Can you work these out from the model? Positions are in its coordinate system, mm. Give positions to 0.01 mm unless a question says otherwise; leave off trailing zeros. Loops run counter-clockwise (first coordinate to the right, second up) from the corner with the lowest first, then second, coordinate; pieces in that order, holes last.
from build123d import *

# Parameters (mm, degrees)
F1_DEPTH    = 86.19552
F3_DEPTH    = 86.19652
F4_T1_DEPTH = 131.920043526


# Not quite as in the source:
# - a fillet or chamfer that OpenCascade refuses, or shapes differently, is made with other operations: its cross-section is extruded or revolved along the edge and cut away or added


with BuildPart() as f1:
    # F0 (on Front) → F1 (new body)
    with BuildSketch(Plane.XZ):
        Polygon((7.1333632804, 110.441185534), (0, 110.441185534), (0, 0), (62.41620332, 0), (62.41620332, 7.1333632804), (7.1333632804, 7.1333632804), align=None)
    extrude(amount=-F1_DEPTH)

    # F2 (on face) → F3 (cut, through all)
    with BuildSketch(Plane.XZ):
        Polygon((7.1333632804, 110.441185534), (7.1333632804, 7.1333632804), (25.2087078989, 24.2729913443), (25.2087078989, 110.441185534), align=None)
        Polygon((2.0419980865, 110.441185534), (7.1333632804, 7.1333632804), (7.1333632804, 110.441185534), align=None)
    extrude(amount=-F3_DEPTH, mode=Mode.SUBTRACT)

    # F4: chamfer of 8.89 on 1 edges, made by hand

    # F4_s2 → F4_t1 (cut)
    with BuildSketch(Plane.XZ.offset(-109.057781763)):
        Polygon((53.52620332, 7.1333632804), (62.41620332, -1.7566367196), (62.41620332, 7.1333632804), align=None)
    extrude(amount=F4_T1_DEPTH, mode=Mode.SUBTRACT)


solid = f1.part
(1) Please list where these lines run through material, in increasing order: probe 1 along Z at (x, y) = (38, 59.5); probe 2 along X at (y, z) = (63, 25); probe 3 along X at (y, z) = (28.5, 68).
Returned:
probe 1: z = 0 to 7.13
probe 2: x = 0 to 6.25
probe 3: x = 0 to 4.13
(2) Thinking about a two-plate mould opening in Z: for faces 1 (the flat face through (5, 86.196, 27)), 2 (the flat face through (30, 42, 0)), 3 (the flat face through (31, 42, 7.133)), which applies, pulls with the +Z half, pulls with the -Z half, needs draft (parallel to the pull), parting line crosses it, or undercut?
Returned:
face 1: needs draft
face 2: pulls with the -Z half
face 3: pulls with the +Z half
(3) Suppose I cut it at C-C on z = 71. List the corners of the cut face in (x, y) for me, plus the area to 3 significant figures.
Returned:
outline: (0, 0) - (3.99, 0) - (3.99, 86.2) - (0, 86.2) - close
area: 344 mm2
(4) Suppose I cut it at A-A on y = 33. List the corners of the cut face in (x, z) for me, plus the area to 3 significant figures.
Returned:
outline: (0, 0) - (60.66, 0) - (53.53, 7.13) - (7.13, 7.13) - (2.04, 110.44) - (0, 110.44) - close
area: 881 mm2
(5) Suppose I cut it at B-B on x = 25. List the corners of the cut face in (y, z) for me.
Returned:
outline: (0, 0) - (86.2, 0) - (86.2, 7.13) - (0, 7.13) - close
(6) Will these pins go through, and if not, where does the flat tip stop? P1, Ø12, axis at x = 37.5, y = 59.5, coming from the +Z side; P2, Ø8, axis at y = 70.5, z = 77.5, coming from the +X side; P3, Ø6, axis at x = 8.5, z = 63.5, coming from the +Y side (3 decimals).
Returned:
P1: stops at z = 7.13
P2: stops at x = 3.86
P3: passes through
